Work out the finished part from the listing and answer in its coordinate system (mm). A direction names the side the tool comes from. Coordinates: 2 decimals unless noted, no trailing zeros. Loops run counter-clockwise (first coordinate to the right, second up) from the corner with the lowest first, then second, coordinate; pieces in that order, holes last.
```python
from build123d import *

# Parameters (mm, degrees)
ESQUISSE1_W             = 1.5
ESQUISSE1_H             = 14
ENL_V_START             = -1.5
ENL_V_MAT_EXTRU_1_DEPTH = 1.5
ENL_V_MAT_EXTRU_2_DEPTH = 1.5
CHANFREIN1_SIZE         = 0.1
CHANFREIN2_SIZE         = 0.1


# Read off the part's stored shape, not the designer's step: Enl_v. mat.-Extru.2
with BuildPart() as part:
    # Esquisse1 → R_volution1 (revolve)
    with BuildSketch(Plane(origin=(0, 0, 10.4), x_dir=(-1, 0, 0), z_dir=(0, 0, -1)), mode=Mode.PRIVATE) as r_volution1_sk:
        with Locations((-1.607807721, -5.637142552)):
            Rectangle(ESQUISSE1_W, ESQUISSE1_H)
    revolve(r_volution1_sk.sketch.rotate(Axis((0.857807721, -12.637142552, 10.4), (0, 1, 0)), 270), axis=Axis((0.857807721, -12.637142552, 10.4), (0, 1, 0)))

    # Esquisse2 → Enl_v. mat.-Extru.1 (cut)
    with BuildSketch(Plane(origin=(0, 1.362857448, 0), x_dir=(-1, 0, 0), z_dir=(0, 1, 0)).offset(ENL_V_START)):
        with BuildLine():
            Line((-2.12666531, 11.2), (0.411050198, 11.2))
            ThreePointArc((0.411050198, 11.2), (-0.857807556, 11.9), (-2.12666531, 11.2))
        make_face()
    extrude(amount=ENL_V_MAT_EXTRU_1_DEPTH, mode=Mode.SUBTRACT)

    # Enl_v. mat.-Extru.2 outline → Enl_v. mat.-Extru.2 (cut)
    with BuildSketch(Plane.XZ.offset(12.637142552).offset(ENL_V_START)):
        with BuildLine():
            ThreePointArc((2.126665453, 11.200000035), (0.85780768, 11.9), (-0.411050055, 11.199999965))
            Line((-0.411050055, 11.199999965), (2.126665453, 11.200000035))
        make_face()
    extrude(amount=ENL_V_MAT_EXTRU_2_DEPTH, mode=Mode.SUBTRACT)

    # Chanfrein1
    chanfrein1_edges = [part.edges().sort_by_distance(p)[0] for p in [
        (0.857807808, 1.362857448, 8.9),
    ]]
    chamfer(chanfrein1_edges, length=CHANFREIN1_SIZE)

    # Chanfrein2
    chanfrein2_edges = [part.edges().sort_by_distance(p)[0] for p in [
        (0.857807762, -12.637142552, 8.9),
    ]]
    chamfer(chanfrein2_edges, length=CHANFREIN2_SIZE)


solid = part.part
```
1. For faces 1 (the flat face through (1, -12, 11.2)), 2 (the cylindrical face through (-0.055, -5.541, 9.21)), 3 (the flat face through (1, 1, 11.2)), determine the directions among +Z, -Z, +X, -X, +Y, -Y from which every point of the face is accessible in a straight line to the end or side of a thin tool.
2. A cutting plane is placed at A-A, the plane y = 0. Give the vertices of the cut face in (x, z).
3. A cutting plane is placed at B-B, the plane y = -4.75. Give the vertices of the cut face in (x, z).
4. Each of these flat-tipped pins is pushed along its axis until it touches: P1, Ø1.6, axis at x = 1, y = 1, coming from the +Z side; P2, Ø0.8, axis at x = 1, z = 11.5, coming from the -Y side. Where does it stop, or does it pass through?
5. Straight lines are drawn through the part: probe 1 along X at (y, z) = (-4.25, 10.3); probe 2 along Y at (x, z) = (1, 11.5); probe 3 along Z at (x, y) = (1.4, 0.25). For each, find the intervals that lie inside material, in ascending order.
Answers below:
1. face 1: +Z, +X, -X, -Y
1. face 2: +Y, -Y
1. face 3: +Z, +X, -X, +Y
2. outline: (-0.41, 11.2) arc R1.5 ccw (long way) to (2.13, 11.2) - close
3. outline: circle Ø3 at (0.86, 10.4)
4. P1: stops at z = 11.2
4. P2: stops at y = -12.64
5. probe 1: x = -0.64 to 2.35
5. probe 2: y = -11.14 to -0.14
5. probe 3: z = 9 to 11.2
